```python
from build123d import *

# Parameters (mm, degrees)
F1_DEPTH = 20
F2_R     = 1
F4_DEPTH = 10
F5_R     = 1


with BuildPart() as f1:
    # F0 (on Top) → F1 (new body)
    with BuildSketch(Plane.XY):
        with BuildLine():
            Line((2.302716, 2), (9.797959, 2))
            ThreePointArc((9.797959, 2), (-10, 0), (9.797959, -2))
            Line((9.797959, -2), (2.302716, -2))
            ThreePointArc((2.302716, -2), (-3.05, 0), (2.302716, 2))
        make_face()
    extrude(amount=F1_DEPTH)

    # F2
    f2_edges = [f1.edges().sort_by_distance(p)[0] for p in [
        (9.797959, 2, 10),
        (2.302716, 2, 10),
        (2.302716, -2, 10),
        (9.797959, -2, 10),
    ]]
    fillet(f2_edges, radius=F2_R)

    # F3 (on Top) → F4 (join)
    with BuildSketch(Plane.XY):
        with BuildLine():
            Line((2.655654, 1.5), (9.88686, 1.5))
            ThreePointArc((9.88686, 1.5), (-10, 0), (9.88686, -1.5))
            Line((9.88686, -1.5), (2.655654, -1.5))
            ThreePointArc((2.655654, -1.5), (-3.05, 0), (2.655654, 1.5))
        make_face()
    extrude(amount=F4_DEPTH)

    # F5
    f5_edges = [f1.edges().sort_by_distance(p)[0] for p in [
        (9.88686, -1.5, 5),
        (9.88686, 1.5, 5),
        (2.655654, -1.5, 5),
        (2.655654, 1.5, 5),
    ]]
    fillet(f5_edges, radius=F5_R)


solid = f1.part
```
The model under review builds one solid part; all positions refer to its coordinate system, in mm. A direction names the side the tool comes from. Give positions to 0.01 mm unless a question says otherwise; leave off trailing zeros. Write each loop counter-clockwise with the first axis right and the second up, starting at its lowest first coordinate (ties: lowest second). Pieces come first, ordered by that corner, then holes.
(1) Consider section B-B, the plane z = 10.75. Give the boundary of the cut face in (x, y).
(2) Consider section C-C, the plane y = 6. Give the boundary of the cut face in (x, z), and give its area (3 significant figures).
(3) Consider section D-D, the plane x = -2. Give the boundary of the cut face in (y, z), and give its area (3 significant figures).
(4) Consider section A-A, the plane x = 0. Give the boundary of the cut face in (y, z).
(5) The part is to be moulded in two halves that separate along Y. For faces 1 (the flat face through (6, 1.5, 5)), 2 (the flat face through (-3, -2, 20)), 3 (the flat face through (6.4, 1.7, 10)), say which applies: released by +Y, released by -Y, zero draft, split by the parting line, or undercut.
(6) To check wall thickness, follow L1, parallel to Y at x = 0, z = 3; L2, parallel to Y at x = 6, z = 5.25; L3, parallel to X at y = 0, z = 7. State the ranges of each line that lie inside material, in increasing order.
(7) For P1, Ø4, axis at x = -0.5, y = 8, coming from the -Z side; P2, Ø2, axis at x = 4.5, z = 8, coming from the +Y side; P3, Ø3, axis at x = 5.5, z = 15.5, coming from the -Y side; P4, Ø6.5, axis at x = 7, z = 15.5, coming from the +Y side, all flat-tipped, find the tip position at first contact; note any pin that passes through.
(8) Tool access review of faces 4 (the cylindrical face through (9.309, -2.434, 15.07)), 5 (the flat face through (-2.5, -2.1, 0)), 6 (the flat face through (6, -1.5, 5)): name each direction out of +Z, -Z, +X, -X, +Y, -Y from which nothing blocks a thin tool from reaching the whole face with its end or side.
Returned:
1. outline: (2.05, -2.26) arc R3.05 cw (long way) to (2.05, 2.26) arc R1 ccw to (2.72, 2) - (8.49, 2) arc R1 ccw to (9.43, 3.33) arc R10 ccw (long way) to (9.43, -3.33) arc R1 ccw to (8.49, -2) - (2.72, -2) arc R1 ccw to start
2. outline: (-8, 0) - (8, 0) - (8, 20) - (-8, 20) - close
2. area: 320 mm2
3. outline: (-9.8, 0) - (-2.3, 0) - (-2.3, 20) - (-9.8, 20) - close; (2.3, 0) - (9.8, 0) - (9.8, 20) - (2.3, 20) - close
3. area: 300 mm2
4. outline: (-10, 0) - (-3.05, 0) - (-3.05, 20) - (-10, 20) - close; (3.05, 0) - (10, 0) - (10, 20) - (3.05, 20) - close
5. face 1: undercut
5. face 2: zero draft
5. face 3: undercut
6. L1: y = -10 to -3.05, 3.05 to 10
6. L2: y = -8 to -1.5, 1.5 to 8
6. L3: x = -10 to -3.05
7. P1: stops at z = 0
7. P2: stops at y = 9.37
7. P3: stops at y = -9.17
7. P4: stops at y = 9.27
8. face 4: +Z, +X
8. face 5: -Z, +X, -X, +Y, -Y
8. face 6: +Z, -Z, +X
